from build123d import *

# Parameters (mm, degrees)
F1_DEPTH = 12.7
F3_DEPTH = 12.701
F5_DEPTH = 12.701


# Not quite as in the source:
# - a length typed as a fraction of an inch, garbled in the dataset ("3 / 203.2 mm" for 3/8 in), is restored


with BuildPart() as f1:
    # F0 (on Right) → F1 (new body)
    with BuildSketch(Plane.YZ):
        Polygon((-313.2666666667, 601.1333333333), (-364.0666666667, 651.9333333333), (-364.0666666667, -364.0666666667), (651.9333333333, -364.0666666667), (601.1333333333, -313.2666666667), (-211.6666666667, -211.6666666667), align=None)
    extrude(amount=F1_DEPTH)

    # F2 (on face) → F3 (cut, through all)
    with BuildSketch(Plane.YZ.offset(12.7)):
        Polygon((-283.3765386061, -292.3567947272), (-287.8666666667, -287.8666666667), (-292.3567947272, -283.3765386061), (-364.0666666667, -355.0864105456), (-364.0666666667, -364.0666666667), (-355.0864105456, -364.0666666667), align=None)
    extrude(amount=-F3_DEPTH, mode=Mode.SUBTRACT)

    # F4 (on face) → F5 (cut, through all)
    with BuildSketch(Plane.YZ.offset(12.7)):
        Polygon((-334.1487050056, -364.0666666667), (-364.0666666667, -334.1487050056), (-364.0666666667, -355.0864105456), (-355.0864105456, -364.0666666667), align=None)
    extrude(amount=-F5_DEPTH, mode=Mode.SUBTRACT)


solid = f1.part
Read the model definition and answer for the solid it produces. Units are mm, in the model's axes. A direction names the side the tool comes from. Give positions to 0.01 mm unless a question says otherwise; leave off trailing zeros. Write each loop counter-clockwise with the first axis right and the second up, starting at its lowest first coordinate (ties: lowest second). Pieces come first, ordered by that corner, then holes. Notation, with made-up numbers: (34, 26) - (54, 26) arc R23 ccw to (54, 59) - close; hole circle Ø11 at (56.25, -23). An arc over 180 degrees is marked (long way). Use CSV: the item, a comma, the result in double quotes. Start each with the question number.
(1) Consider line 1 along Y through (x, z) = (3, 63); line 2 along Z through (x, y) = (1, -106) (3 decimals); line 3 along Z through (x, y) = (4.5, -133.5). Determine where each line is inside the solid, lowest interval first.
(2) Given P1, Ø6, axis at x = 10, z = 100.5, coming from the +Y side; P2, Ø3, axis at x = 5.5, y = 33.5, coming from the +Z side (3 decimals), each flat-ended and moving along its own axis, determine where each tip first touches the part or whether it passes through.
(3) Determine the mould class of faces 3 (the flat face through (6.261, -261.755, 189.044)), 4 (the flat face through (0, -235, -117)), 5 (the flat face through (6.44, -322.55, -313.57)) for opening direction Y: +Y half, -Y half, draft (parallel to the pull), parting line (faces both ways), or undercut.
(4) Find section A-A (x = 2.5). Give the vertices of the cut face in (y, z), plus the area to 3 significant figures.
(5) Find section C-C (y = 35). Give the vertices of the cut face in (x, z), plus the area to 3 significant figures.
(6) For faces 1 (the flat face through (6.44, -314.43, -323.41)), 2 (the flat face through (6.261, -338.311, 626.178)), determine the directions among +Z, -Z, +X, -X, +Y, -Y from which every point of the face is accessible in a straight line to the end or side of a thin tool.
(7) Find section B-B (z = 569). Give the vertices of the cut face in (x, y), plus the area to 3 significant figures.
Findings below:
1,line 1,"-364.07 to -246"
1,line 2,"-364.067 to -224.875"
1,line 3,"-364.07 to -221.44"
2,P1,"y = -250.31"
2,P2,"z = -242.125"
3,face 3,"+Y half"
3,face 4,"draft"
3,face 5,"undercut"
4,outline,"(-364.07, -334.15) - (-353.6, -344.62) - (-292.36, -283.38) - (-283.38, -292.36) - (-344.62, -353.6) - (-334.15, -364.07) - (651.93, -364.07) - (601.13, -313.27) - (-211.67, -211.67) - (-313.27, 601.13) - (-364.07, 651.93) - close"
4,area,"189,000 mm2"
5,outline,"(0, -364.07) - (12.7, -364.07) - (12.7, -242.5) - (0, -242.5) - close"
5,area,"1,540 mm2"
6,face 1,"+X, -X"
6,face 2,"+Z, +X, -X, +Y"
7,outline,"(0, -364.07) - (12.7, -364.07) - (12.7, -309.25) - (0, -309.25) - close"
7,area,"696 mm2"
